Model file for the job. Use its own axes, mm. Face numbers are marked on the shaded views. A direction names the side the tool comes from. Round coordinates to 2 decimals unless told otherwise and drop trailing zeros. Write each loop counter-clockwise with the first axis right and the second up, starting at its lowest first coordinate (ties: lowest second). Pieces come first, ordered by that corner, then holes.
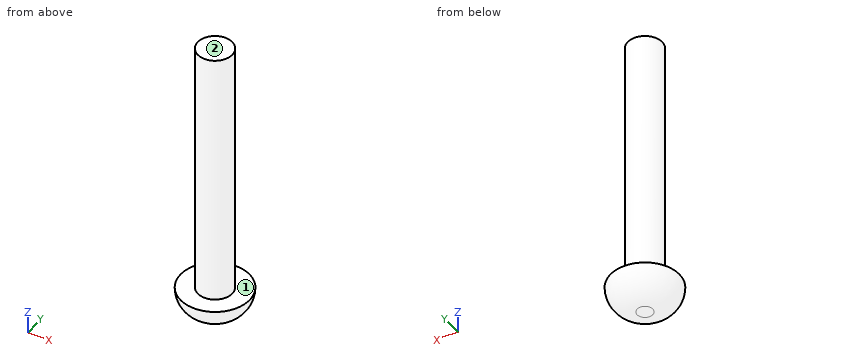
Autodesk Inventor part; units mm, degrees
ref_plane "YZ Plane" through (0, 0, 0) normal (1, 0, 0) x (0, 1, 0)
ref_plane "XZ Plane" through (0, 0, 0) normal (0, 1, 0) x (-1, 0, 0)
ref_plane "XY Plane" through (0, 0, 0) normal (0, 0, 1) x (1, 0, 0)
sketch "スケッチ1" plane through (0, 0, 0) normal (0, 0, 1) x (1, 0, 0)
  circle A0 centre (0, 0) radius 2
  dimension "d1" = 4
extrude "押し出し1" add sketch "スケッチ1" along normal blind 30
sketch "スケッチ2" plane through (0, 0, 0) normal (0, 0, -1) x (-1, 0, 0)
  circle A0 centre (0, 0) radius 2
  circle A1 centre (0, 0) radius 4
  dimension "d4" = 8
extrude "押し出し2" add sketch "スケッチ2" along normal blind 3.1 contours A0 | A1
fillet "フィレット1" radius 3.1 1 edges at (4, 0, -3.1)
thread "ねじ1"
properties part number "ネジ鍋m4,30" material "鋼、高強度、低合金"
1) Which spindle directions (+Z, -Z, +X, -X, +Y, -Y) get a long thin tool onto all of the face, cutting with end or side? Do the marked faces 1 and 2. Say none if no direction does.
2) Cut at A-A on z = 27. List the corners of the cut face in (x, y), and give its area (3 significant figures).
3) Flat gauge pins, fed straight in: pin 1 Ø1 at (y, z) = (-1.5, 3) entering from +X; pin 2 Ø2 at (x, z) = (-2, 13) entering from +Y; pin 3 Ø2 at (x, y) = (-3, 3) entering from +Z. Where does each tip first touch, or does it go through?
4) Wall check: probe 1 along Y at (x, z) = (0, 19); probe 2 along Z at (x, y) = (-2.5, 2.5); probe 3 along Y at (x, z) = (-0.5, 8). Give the ranges that are in metal, low to high.
Result sheet:
1. face 1: +Z
1. face 2: +Z, +X, -X, +Y, -Y
2. outline: circle Ø4 at (0, 0)
2. area: 12.6 mm2
3. pin 1: stops at x = 1.73
3. pin 2: stops at y = 1.73
3. pin 3: stops at z = 0
4. probe 1: y = -2 to 2
4. probe 2: z = -1.63 to 0
4. probe 3: y = -1.94 to 1.94
